Read the model definition and answer for the solid it produces. Units are mm, in the model's axes. Face numbers are marked on the shaded views. A direction names the side the tool comes from. Give positions to 0.01 mm unless a question says otherwise; leave off trailing zeros. Loops run counter-clockwise (first coordinate to the right, second up) from the corner with the lowest first, then second, coordinate; pieces in that order, holes last.
(1) Each of these flat-tipped pins is pushed along its axis until it touches: P1, Ø4, axis at x = 5.5, z = -12.5, coming from the +Y side; P2, Ø12, axis at y = 33, z = -17, coming from the -X side; P3, Ø1.5, axis at x = 2.5, z = -13.5, coming from the -Y side; P4, Ø6, axis at x = 3.5, y = 18, coming from the +Z side. Where does it stop, or does it pass through?
(2) Which of the six approach directions +Z, -Z, +X, -X, +Y, -Y give full straight-line access (tool end or side, diameter ignored) to the marked faces 1, 2 and 3?
(3) Straight lines are drawn through the part: probe 1 along X at (y, z) = (36.5, -27); probe 2 along X at (y, z) = (14.5, -19); probe 3 along Z at (x, y) = (11.25, 37.5). For each, find the intervals that lie inside material, in ascending order.
(4) Find section B-B, the plane z = -28. Write down the section's boundary in (x, y), then the cut area to 3 significant figures.
(5) Find section D-D, the plane z = -21. Write down the section's boundary in (x, y).
(6) Find section C-C, the plane y = 4. Write down the section's boundary in (x, z).
(7) Find section A-A, the plane x = 7. Write down the section's boundary in (y, z), then the cut area to 4 significant figures.
(8) Determine the mould class of the marked faces 4, 5 and 6 for opening direction Z: pulls with the +Z half, pulls with the -Z half, needs draft (parallel to the pull), parting line crosses it, or undercut.
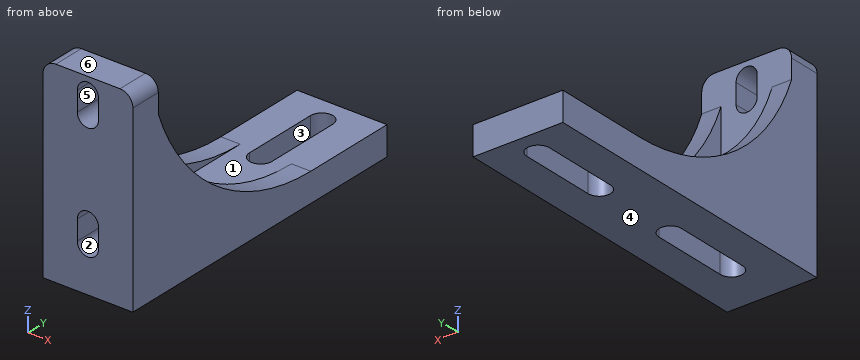
```python
from build123d import *

# Parameters (mm, degrees)
CROQUIS2_W              = 14
CROQUIS2_H              = 31
CROQUIS2_R              = 1.55
SALIENTE_EXTRUIR1_DEPTH = 50
CROQUIS3_W              = 26
CROQUIS3_H              = 45
CORTAR_EXTRUIR1_DEPTH   = 14
CORTAR_EXTRUIR2_DEPTH   = 5
SALIENTE_EXTRUIR3_DEPTH = 14
CROQUIS7_OUTSIDE_W      = 28.094
CROQUIS7_OUTSIDE_H      = 45.094
CORTAR_EXTRUIR5_DEPTH   = 45
REDONDEO1_R             = 2
CROQUIS8_W              = 14
CROQUIS8_H              = 0.5
CORTAR_EXTRUIR6_DEPTH   = 50
CORTAR_EXTRUIR7_DEPTH   = 5


with BuildPart() as part:
    # Croquis2 → Saliente-Extruir1 (new body)
    with BuildSketch(Plane(origin=(0, 0, 0), x_dir=(1, 0, 0), z_dir=(0, 1, 0))):
        with Locations((7, 15.5)):
            Rectangle(CROQUIS2_W, CROQUIS2_H)
        with Locations((7, 22)):
            Circle(CROQUIS2_R, mode=Mode.SUBTRACT)
        with Locations((7, 4)):
            Circle(CROQUIS2_R, mode=Mode.SUBTRACT)
    extrude(amount=SALIENTE_EXTRUIR1_DEPTH)

    # Croquis3 → Cortar-Extruir1 (cut)
    with BuildSketch(Plane.ZY):
        with Locations((-13, 27.5)):
            Rectangle(CROQUIS3_W, CROQUIS3_H)
    extrude(amount=-CORTAR_EXTRUIR1_DEPTH, mode=Mode.SUBTRACT)

    # Croquis4 → Cortar-Extruir2 (cut)
    with BuildSketch(Plane(origin=(0, 0, -31), x_dir=(-1, 0, 0), z_dir=(0, 0, -1))):
        with BuildLine():
            Line((-8.75, 8), (-8.75, 20))
            ThreePointArc((-8.75, 20), (-7, 21.75), (-5.25, 20))
            Line((-5.25, 20), (-5.25, 8))
            ThreePointArc((-5.25, 8), (-7, 6.25), (-8.75, 8))
        make_face()
        with BuildLine():
            Line((-8.75, 34), (-8.75, 46))
            ThreePointArc((-8.75, 46), (-7, 47.75), (-5.25, 46))
            Line((-5.25, 46), (-5.25, 34))
            ThreePointArc((-5.25, 34), (-7, 32.25), (-8.75, 34))
        make_face()
    extrude(amount=-CORTAR_EXTRUIR2_DEPTH, mode=Mode.SUBTRACT)

    # Croquis6 → Saliente-Extruir3 (add)
    with BuildSketch(Plane.ZY):
        with BuildLine():
            Line((-26, 5), (-26, 35))
            ThreePointArc((-26, 35), (-20.21590319, 16.698867767), (-5, 5))
            Line((-5, 5), (-26, 5))
        make_face()
    extrude(amount=-SALIENTE_EXTRUIR3_DEPTH)

    # Croquis7 outside → Cortar-Extruir5 (cut)
    with BuildSketch(Plane(origin=(0, 50, 0), x_dir=(1, 0, 0), z_dir=(0, 1, 0))):
        with Locations((7, 15.5)):
            Rectangle(CROQUIS7_OUTSIDE_W, CROQUIS7_OUTSIDE_H)
        Polygon((0, 26), (0, 0), (3, 0), (3, 26), (11, 26), (11, 0), (14, 0), (14, 26), (14, 31), (0, 31), align=None, mode=Mode.SUBTRACT)
    extrude(amount=-CORTAR_EXTRUIR5_DEPTH, mode=Mode.SUBTRACT)

    # Redondeo1
    redondeo1_edges = [part.edges().sort_by_distance(p)[0] for p in [
        (14, 2.5, 0),
        (0, 2.5, 0),
    ]]
    fillet(redondeo1_edges, radius=REDONDEO1_R)

    # Croquis8 → Cortar-Extruir6 (cut)
    with BuildSketch(Plane(origin=(0, 50, 0), x_dir=(1, 0, 0), z_dir=(0, 1, 0))):
        with Locations((7, 30.75)):
            Rectangle(CROQUIS8_W, CROQUIS8_H)
    extrude(amount=-CORTAR_EXTRUIR6_DEPTH, mode=Mode.SUBTRACT)

    # Croquis9 → Cortar-Extruir7 (cut)
    with BuildSketch(Plane.XZ):
        with BuildLine():
            Line((8.65, -20.45), (8.65, -23.55))
            ThreePointArc((8.65, -23.55), (7, -25.2), (5.35, -23.55))
            Line((5.35, -23.55), (5.35, -20.45))
            ThreePointArc((5.35, -20.45), (7, -18.8), (8.65, -20.45))
        make_face()
        with BuildLine():
            Line((8.65, -2.45), (8.65, -5.55))
            ThreePointArc((8.65, -5.55), (7, -7.2), (5.35, -5.55))
            Line((5.35, -5.55), (5.35, -2.45))
            ThreePointArc((5.35, -2.45), (7, -0.8), (8.65, -2.45))
        make_face()
    extrude(amount=-CORTAR_EXTRUIR7_DEPTH, mode=Mode.SUBTRACT)


solid = part.part
```
Entries:
1. P1: stops at y = 5
1. P2: passes through
1. P3: stops at y = 0
1. P4: stops at z = -18.97
2. face 1: +Z, +Y
2. face 2: +Y, -Y
2. face 3: +Z, -Z
3. probe 1: x = 0 to 5.25, 8.75 to 14
3. probe 2: x = 0 to 3, 11 to 14
3. probe 3: z = -30.5 to -26
4. outline: (0, 0) - (14, 0) - (14, 50) - (0, 50) - close; hole (5.25, 8) arc R1.75 ccw to (8.75, 8) - (8.75, 20) arc R1.75 ccw to (5.25, 20) - close; hole (5.25, 34) arc R1.75 ccw to (8.75, 34) - (8.75, 46) arc R1.75 ccw to (5.25, 46) - close
4. area: 597 mm2
5. outline: (0, 0) - (5.35, 0) - (5.35, 5) - (3, 5) - (3, 17.87) - (0, 17.87) - close; (8.65, 0) - (14, 0) - (14, 17.87) - (11, 17.87) - (11, 5) - (8.65, 5) - close
6. outline: (0, -30.5) - (14, -30.5) - (14, -2) arc R2 ccw to (12, 0) - (2, 0) arc R2 ccw to (0, -2) - close; hole (5.35, -23.55) arc R1.65 ccw to (8.65, -23.55) - (8.65, -20.45) arc R1.65 ccw to (5.35, -20.45) - close; hole (5.35, -5.55) arc R1.65 ccw to (8.65, -5.55) - (8.65, -2.45) arc R1.65 ccw to (5.35, -2.45) - close
7. outline: (0, -30.5) - (6.25, -30.5) - (6.25, -26) - (5, -26) - (5, -25.2) - (0, -25.2) - close; (0, -18.8) - (5, -18.8) - (5, -7.2) - (0, -7.2) - close; (0, -0.8) - (5, -0.8) - (5, 0) - (0, 0) - close; (21.75, -30.5) - (32.25, -30.5) - (32.25, -26) - (21.75, -26) - close; (47.75, -30.5) - (50, -30.5) - (50, -26) - (47.75, -26) - close
7. area: 151.5 mm2
8. face 4: pulls with the -Z half
8. face 5: undercut
8. face 6: pulls with the +Z half
